Autodesk Inventor part; units mm, degrees
ref_plane "YZ Plane" through (0, 0, 0) normal (1, 0, 0) x (0, 1, 0)
ref_plane "XZ Plane" through (0, 0, 0) normal (0, 1, 0) x (-1, 0, 0)
ref_plane "XY Plane" through (0, 0, 0) normal (0, 0, 1) x (1, 0, 0)
sketch "Sketch1" plane through (0, 0, 0) normal (0, 0, 1) x (1, 0, 0)
  line L0 (0, 0) -> (51, 0)
  line L1 (51, 0) -> (51, 16)
  line L2 (51, 16) -> (0, 16)
  line L3 (0, 16) -> (0, 0)
  line L4 (25.5, 0) -> (25.5, 7.5) construction
  line L5 (25.5, 0) -> (25.5, 10.5) construction
  circle A0 centre (25.5, 10.5) radius 4
  dimension "d0" = 51
  dimension "d1" = 16
  dimension "d4" = 10.5
  dimension "d8" = 8
extrude "Extrusion1" add sketch "Sketch1" along normal blind 8 contours L3 L2 L1 L0 | A0
sketch "Sketch2" plane through (0, 0, 0) normal (0, 0, -1) x (-1, 0, 0)
  line L0 (0, 0) -> (-51, 0) construction
  line L1 (-25.5, 0) -> (-25.5, 10.5) construction
  circle A0 centre (-25.5, 10.5) radius 4.75
  line L2 (-25.5, 0) -> (-15.5, 0) construction
  line L3 (-15.5, 0) -> (-15.5, 10.5) construction
  line L4 (-25.5, 0) -> (-35.5, 0) construction
  line L5 (-35.5, 0) -> (-35.5, 10.5) construction
  circle A1 centre (-35.5, 10.5) radius 3
  circle A2 centre (-15.5, 10.5) radius 3
  dimension "d6" = 10.5
  dimension "d7" = 9.5
  dimension "d11" = 10
  dimension "d12" = 10.5
  dimension "d13" = 10
  dimension "d14" = 10.5
  dimension "d15" = 6
  dimension "d16" = 6
extrude "Extrusion2" cut sketch "Sketch2" against normal blind 3 contours A0
sketch "Sketch3" plane through (0, 0, 8) normal (0, 0, 1) x (1, 0, 0)
  line L0 (51, 16) -> (0, 16) construction
  line L1 (0, 16) -> (5, 16) construction
  line L2 (5, 16) -> (5, 11) construction
  point P0 (0, 0)
  dimension "d17" = 5
  dimension "d18" = 5
sketch "Sketch4" plane through (0, 0, 8) normal (0, 0, 1) x (1, 0, 0)
  line L0 (51, 16) -> (0, 16)
  line L1 (0, 16) -> (0, 11)
  line L2 (0, 16) -> (0, 0)
  line L3 (0, 11) -> (5, 11)
  line L4 (51, 16) -> (46, 16)
  line L5 (46, 16) -> (46, 11)
  dimension "d19" = 5
  dimension "d20" = 5
  dimension "d21" = 5
  dimension "d22" = 5
hole "Hole1" at (5, 11, 8) at (46, 11, 8) direction (0, 0, -1) diameter 2.4 end through all counterbore diameter 4.4 counterbore depth 2
sketch "Sketch5" plane through (0, 0, 8) normal (0, 0, 1) x (1, 0, 0)
  point P0 (0, 0)
properties part number "Back Plate" material "Steel, Carbon"
Check sheet for the modelled part. Datum: model origin and axes. Units: mm. A direction names the side the tool comes from. Coordinates: 2 decimals unless noted, no trailing zeros. Loops run counter-clockwise (first coordinate to the right, second up) from the corner with the lowest first, then second, coordinate; pieces in that order, holes last.
1) Material ranges on probe 1 along X at (y, z) = (11, 7.1); probe 2 along Y at (x, z) = (46, 2.35); probe 3 along Y at (x, z) = (46, 6.8), recorded low to high.
2) Sectioned sample at D-D (x = 25.5). Record the boundary of the cut face in (y, z).
3) Sectioned sample at B-B (z = 1). Record the boundary of the cut face in (x, y).
4) Sectioned sample at A-A (x = 46). Record the boundary of the cut face in (y, z), and give its area (3 significant figures).
5) Access from +Z, -Z, +X, -X, +Y, -Y to the whole of each face (thin tool, end or side, straight path). Record for faces 1 (the face through (6, 10, 6)), 2 (the face through (25, 8, 8)), 3 (the face through (26, 11, 3)).
6) Release check for a two-part mould opening along X. For faces 4 (the face through (47, 10, 6)), 5 (the face through (5.843, 8.968, 6.986)), 6 (the face through (51, 8, 4)), 7 (the face through (0, 8, 4)) record: released by +X, released by -X, zero draft, split by the parting line, or undercut.
7) Sectioned sample at C-C (y = 11). Record the boundary of the cut face in (x, z).
8) Gauge pin test, flat ends, axial feed: pin 1 (3 mm diameter, centred on x = 5, y = 11, fed in from +Z); pin 2 (3 mm diameter, centred on x = 25.5, y = 10.5, fed in from -Z). Record the tip position at first contact, or that the pin passes through.
Check sheet entries:
1. probe 1: x = 0 to 2.8, 7.2 to 43.8, 48.2 to 51
1. probe 2: y = 0 to 9.8, 12.2 to 16
1. probe 3: y = 0 to 8.8, 13.2 to 16
2. outline: (0, 0) - (5.75, 0) - (5.75, 3) - (15.25, 3) - (15.25, 0) - (16, 0) - (16, 8) - (0, 8) - close
3. outline: (0, 0) - (51, 0) - (51, 16) - (0, 16) - close; hole circle Ø2.4 at (5, 11); hole circle Ø9.5 at (25.5, 10.5); hole circle Ø2.4 at (46, 11)
4. outline: (0, 0) - (9.8, 0) - (9.8, 6) - (8.8, 6) - (8.8, 8) - (0, 8) - close; (12.2, 0) - (16, 0) - (16, 8) - (13.2, 8) - (13.2, 6) - (12.2, 6) - close
4. area: 105 mm2
5. face 1: +Z
5. face 2: +Z, +X, -X, +Y, -Y
5. face 3: -Z
6. face 4: undercut
6. face 5: undercut
6. face 6: released by +X
6. face 7: released by -X
7. outline: (0, 0) - (3.8, 0) - (3.8, 6) - (2.8, 6) - (2.8, 8) - (0, 8) - close; (6.2, 0) - (20.78, 0) - (20.78, 3) - (30.22, 3) - (30.22, 0) - (44.8, 0) - (44.8, 6) - (43.8, 6) - (43.8, 8) - (7.2, 8) - (7.2, 6) - (6.2, 6) - close; (47.2, 0) - (51, 0) - (51, 8) - (48.2, 8) - (48.2, 6) - (47.2, 6) - close
8. pin 1: stops at z = 6
8. pin 2: stops at z = 3
